```python
from build123d import *

# Parameters (mm, degrees)
SKETCH1_R           = 30
SKETCH1_R_2         = 2.75
BOSS_EXTRUDE1_DEPTH = 3


with BuildPart() as part:
    # Sketch1 → Boss-Extrude1 (new body)
    with BuildSketch(Plane.YZ):
        with Locations(Location((0, 0, 0), (0, 0, 270))):
            Circle(SKETCH1_R)
        with Locations(Location((0, 21.5, 0), (0, 0, 270))):
            Circle(SKETCH1_R_2, mode=Mode.SUBTRACT)
        with Locations(Location((20.4477151, 6.643865379, 0), (0, 0, 270))):
            Circle(SKETCH1_R_2, mode=Mode.SUBTRACT)
        with Locations(Location((12.637382924, -17.393865379, 0), (0, 0, 270))):
            Circle(SKETCH1_R_2, mode=Mode.SUBTRACT)
        with Locations(Location((-12.637382924, -17.393865379, 0), (0, 0, 270))):
            Circle(SKETCH1_R_2, mode=Mode.SUBTRACT)
        with Locations(Location((-20.4477151, 6.643865379, 0), (0, 0, 270))):
            Circle(SKETCH1_R_2, mode=Mode.SUBTRACT)
    extrude(amount=BOSS_EXTRUDE1_DEPTH)


solid = part.part
```
For this review, take the finished solid that the model builds, in its own axes (mm). Coordinates: 2 decimals unless noted, no trailing zeros. Write each loop counter-clockwise with the first axis right and the second up, starting at its lowest first coordinate (ties: lowest second). Pieces come first, ordered by that corner, then holes. Notation, with made-up numbers: (-13.5, 40.25) - (22.5, 40.25) arc R24 ccw to (22.5, 67.25) - close; hole circle Ø9 at (28, 40). An arc over 180 degrees is marked (long way). Answer in a Markdown table with one row per item. Add a question column.
Q1. We need section B-B, the plane z = 21.5. State the section outline as (x, y) points, and give its area (3 significant figures).
Q2. We need section D-D, the plane z = 13.5. State the section outline as (x, y) points, and give its area (3 significant figures).
Q3. We need section A-A, the plane y = 0. State the section outline as (x, z) points.
Q4. Draft analysis for pull direction Z (two halves, no side actions). For faces 1 (the flat face through (0, 0, 0)), 2 (the cylindrical face through (1.48, 1.32, 29.97)), 3 (the cylindrical face through (1.48, 20.57, 9.39)), state which applies: +Z half, -Z half, draft (parallel to the pull), parting line (faces both ways), or undercut.
Q5. For probe 1 along Y at (x, z) = (2.65, -17); probe 2 along Y at (x, z) = (1.15, 6.5); probe 3 along Y at (x, z) = (1.2, 20), list the stretches that pass through material, from the lowest coordinate up.
Q6. For P1, Ø4.5, axis at y = -20.45, z = 6.64, coming from the -X side; P2, Ø1, axis at x = 1.5, z = 11.5, coming from the -Y side; P3, Ø1, axis at x = 1.5, y = 8, coming from the -Z side, all flat-tipped, find the tip position at first contact; note any pin that passes through.
Q7. We need section C-C, the plane x = 2.2. State the section outline as (y, z) points.
Answer list:
| question | item | result |
|---|---|---|
| 1 | outline | (0, -20.92) - (3, -20.92) - (3, -2.75) - (0, -2.75) - close; (0, 2.75) - (3, 2.75) - (3, 20.92) - (0, 20.92) - close |
| 1 | area | 109 mm2 |
| 2 | outline | (0, -26.79) - (3, -26.79) - (3, 26.79) - (0, 26.79) - close |
| 2 | area | 161 mm2 |
| 3 | outline | (0, -30) - (3, -30) - (3, 18.75) - (0, 18.75) - close; (0, 24.25) - (3, 24.25) - (3, 30) - (0, 30) - close |
| 4 | face 1 | draft |
| 4 | face 2 | parting line |
| 4 | face 3 | undercut |
| 5 | probe 1 | y = -24.72 to -15.36, -9.92 to 9.92, 15.36 to 24.72 |
| 5 | probe 2 | y = -29.29 to -23.19, -17.7 to 17.7, 23.19 to 29.29 |
| 5 | probe 3 | y = -22.36 to -2.3, 2.3 to 22.36 |
| 6 | P1 | passes through |
| 6 | P2 | stops at y = -27.91 |
| 6 | P3 | stops at z = -29.05 |
| 7 | outline | circle Ø60 at (0, 0); hole circle Ø5.5 at (-20.45, 6.64); hole circle Ø5.5 at (-12.64, -17.39); hole circle Ø5.5 at (0, 21.5); hole circle Ø5.5 at (12.64, -17.39); hole circle Ø5.5 at (20.45, 6.64) |
